from build123d import *

# Parameters (mm, degrees)
SKETCH_4_W          = 30
SKETCH_4_H          = 65
EXTRUDE_1_DEPTH     = 20
SKETCH_5_W          = 7.9
SKETCH_5_H          = 14.15
CUT_EXTRUDE_1_DEPTH = 8


with BuildPart() as part:
    # 草图4 → 凸台-拉伸1 (new body)
    with BuildSketch(Plane(origin=(0, 0, 0), x_dir=(1, 0, 0), z_dir=(0, 1, 0))):
        Rectangle(SKETCH_4_W, SKETCH_4_H)
    extrude(amount=EXTRUDE_1_DEPTH)

    # 草图5 → 切除-拉伸1 (cut)
    with BuildSketch(Plane(origin=(0, 0, 0), x_dir=(-1, 0, 0), z_dir=(0, -1, 0))):
        with Locations((11.05, -17.425)):
            Rectangle(SKETCH_5_W, SKETCH_5_H)
        with Locations((11.05, 16.225)):
            Rectangle(SKETCH_5_W, SKETCH_5_H)
        with Locations((-11.05, 16.225)):
            Rectangle(SKETCH_5_W, SKETCH_5_H)
        with Locations((-11.05, -17.425)):
            Rectangle(SKETCH_5_W, SKETCH_5_H)
    extrude(amount=-CUT_EXTRUDE_1_DEPTH, mode=Mode.SUBTRACT)


solid = part.part
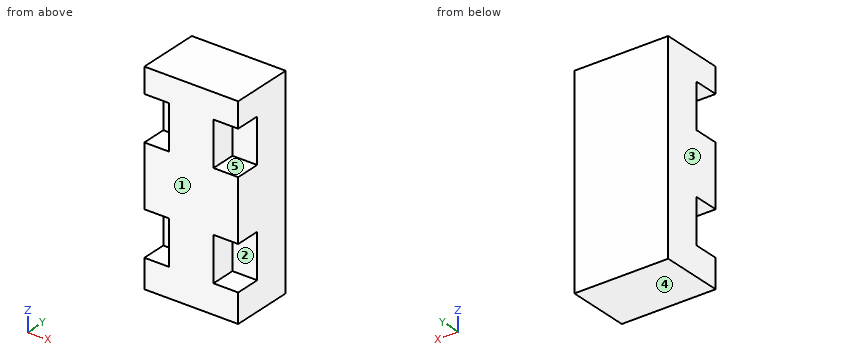
For this review, take the finished solid that the model builds, in its own axes (mm). Face numbers are marked on the shaded views. A direction names the side the tool comes from. Give positions to 0.01 mm unless a question says otherwise; leave off trailing zeros. Loops run counter-clockwise (first coordinate to the right, second up) from the corner with the lowest first, then second, coordinate; pieces in that order, holes last. Notation, with made-up numbers: M -12,37 L 11,37 A28 cw 11,55 Z; hole C 65,22.5 d9. An arc over 180 degrees is marked long. Put each result on its own line as item: value. Start each with the question number.
(1) Add section B-B, the plane x = 10.5. Write out the cut boundary in (y, z).
(2) Wall thickness on L1, parallel to Z at x = -13.5, y = 3.75; L2, parallel to X at y = 7.5, z = 11; L3, parallel to Y at x = -13.5, z = 19.5: over which ranges is each line inside the solid? List them lowest first.
(3) The part is to be moulded in two halves that separate along Z. For the marked faces 3, 4 and 5, say which applies: +Z half, -Z half, draft (parallel to the pull), parting line (faces both ways), or undercut.
(4) For pin 1 (2.5 mm diameter, centred on y = 4, z = -14.5, fed in from +X); pin 2 (2.5 mm diameter, centred on x = 10.5, z = -18, fed in from -Y), all flat-tipped, find the tip position at first contact; note any pin that passes through.
(5) Machinability: for the marked faces 1 and 2, which of the approach directions +Z, -Z, +X, -X, +Y, -Y give a long, thin tool a straight path to every point of the face, cutting with its end or side? Answer none if there is none.
(6) Add section A-A, the plane z = 12. Write out the cut boundary in (x, y), then the cut area to 3 significant figures.
Result:
1. outline: M 0,-32.5 L 20,-32.5 L 20,32.5 L 0,32.5 L 0,24.5 L 8,24.5 L 8,10.35 L 0,10.35 L 0,-9.15 L 8,-9.15 L 8,-23.3 L 0,-23.3 Z
2. L1: z = -32.5 to -23.3, -9.15 to 10.35, 24.5 to 32.5
2. L2: x = -7.1 to 7.1
2. L3: y = 8 to 20
3. face 3: draft
3. face 4: -Z half
3. face 5: undercut
4. pin 1: stops at x = 7.1
4. pin 2: stops at y = 8
5. face 1: +Z, -Z, +X, -X, -Y
5. face 2: +X, -Y
6. outline: M -15,8 L -7.1,8 L -7.1,0 L 7.1,0 L 7.1,8 L 15,8 L 15,20 L -15,20 Z
6. area: 474 mm^2
